```python
from build123d import *

# Parameters (mm, degrees)
POCKET003_DEPTH    = 10
POLARPATTERN_COUNT = 6


with BuildPart() as part:
    # Sketch012 → Revolution001 (revolve)
    with BuildSketch(Plane.XZ):
        Polygon((4, 0), (4, 2.040516), (7.084628, 2.040516), (7.084628, 14), (9, 14), (9, 0), align=None)
    revolve(axis=Axis((0, 0, 0), (0, 0, 1)))

    # Sketch013 → Pocket003 (cut, symmetric)
    with BuildSketch(Plane.XZ):
        with BuildLine():
            ThreePointArc((11.928039, 6.425307), (10.121972, 8.231374), (8.315905, 6.425307))
            Line((8.315905, 6.425307), (8.315905, -3.082439))
            ThreePointArc((8.315905, -3.082439), (10.121972, -4.888506), (11.928039, -3.082439))
            Line((11.928039, 6.425307), (11.928039, -3.082439))
        make_face()
    pocket003 = extrude(amount=POCKET003_DEPTH, both=True, mode=Mode.SUBTRACT)

    # PolarPattern: Pocket003 ×6 about axis
    polarpattern_axis = Axis((0, 0, 0), (0, 0, 1))
    for i in range(1, POLARPATTERN_COUNT):
        add(pocket003.rotate(polarpattern_axis, i * 360 / POLARPATTERN_COUNT), mode=Mode.SUBTRACT)


with BuildPart() as part_1:
    # Body006 placement: moved
    add(part.part.moved(Location((0, 0, -34))))


solid = part_1.part
```
The listing builds one solid part. Answer for the finished solid, in the listing's coordinates (mm). A direction names the side the tool comes from. Round coordinates to 2 decimals unless told otherwise and drop trailing zeros. Loops run counter-clockwise (first coordinate to the right, second up) from the corner with the lowest first, then second, coordinate; pieces in that order, holes last.
Q1. Section D-D, the plane y = 4.75 is taken. Determine the outline of the cut face in (x, z), then the cut area to 3 significant figures.
Q2. Which of the six approach directions +Z, -Z, +X, -X, +Y, -Y give full straight-line access (tool end or side, diameter ignored) to faces 5 (the face through (-8.316, 0, -31)), 6 (the face through (-4.116, 7.226, -30.742)), 7 (the face through (8.316, 0, -31)), 8 (the face through (4.2, 7.178, -30.742))?
Q3. Section C-C, the plane y = 0 is taken. Determine the outline of the cut face in (x, z), then the cut area to 3 significant figures.
Q4. Section B-B, the plane z = -28.25 is taken. Determine the outline of the cut face in (x, y).
Q5. Find the intervals of material crossed by line 1 (Y direction, x = 0, z = -33.35); line 2 (Z direction, x = -6, y = -0.75); line 3 (Y direction, x = 6.5, z = -28.5), in increasing order.
Q6. For a pull along Y with two mould halves and no side action, classify faces 1 (the face through (-0.867, -3.905, -32.965)), 2 (the face through (-4.17, 7.33, -26.94)), 3 (the face through (-4.257, -7.277, -26.941)), 4 (the face through (-3, -3, -31.959)) as released by +Y, released by -Y, zero draft, split by the parting line, or undercut.
Q7. Section A-A, the plane x = 0 is taken. Determine the outline of the cut face in (y, z), then the cut area to 3 significant figures.
Q8. Given pin 1 Ø1.5 at (x, z) = (-4, -23) entering from +Y; pin 2 Ø7 at (y, z) = (-1.5, -31) entering from +X; pin 3 Ø1.5 at (y, z) = (2.5, -24) entering from +X, each flat-ended and moving along its own axis, determine where each tip first touches the part or whether it passes through.
Completed:
1. outline: (-7.64, -34) - (7.64, -34) - (7.64, -20) - (5.26, -20) - (5.26, -31.96) - (-5.26, -31.96) - (-5.26, -20) - (-7.64, -20) - close
1. area: 88.3 mm2
2. face 5: -Z, -X, +Y, -Y
2. face 6: -Z, -X, +Y
2. face 7: -Z, +X, +Y, -Y
2. face 8: -Z, +X, +Y
3. outline: (-9, -26.16) arc R1.81 cw to (-8.32, -27.57) - (-8.32, -34) - (-4, -34) - (-4, -31.96) - (-7.08, -31.96) - (-7.08, -20) - (-9, -20) - close; (4, -34) - (8.32, -34) - (8.32, -27.57) arc R1.81 cw to (9, -26.16) - (9, -20) - (7.08, -20) - (7.08, -31.96) - (4, -31.96) - close
3. area: 56.1 mm2
4. outline: (-8.32, -3.44) arc R9 ccw to (-7.14, -5.48) - (-1.18, -8.92) arc R9 ccw to (1.18, -8.92) - (7.14, -5.48) arc R9 ccw to (8.32, -3.44) - (8.32, 3.44) arc R9 ccw to (7.14, 5.48) - (1.18, 8.92) arc R9 ccw to (-1.18, 8.92) - (-7.14, 5.48) arc R9 ccw to (-8.32, 3.44) - close; hole circle Ø14.17 at (0, 0)
5. line 1: y = -9 to -4, 4 to 9
5. line 2: z = -34 to -31.96
5. line 3: y = -5.85 to -2.82, 2.82 to 5.85
6. face 1: undercut
6. face 2: released by +Y
6. face 3: released by -Y
6. face 4: undercut
7. outline: (-9, -34) - (-4, -34) - (-4, -31.96) - (-7.08, -31.96) - (-7.08, -20) - (-9, -20) - close; (4, -34) - (9, -34) - (9, -20) - (7.08, -20) - (7.08, -31.96) - (4, -31.96) - close
7. area: 66.2 mm2
8. pin 1: stops at y = 8.39
8. pin 2: stops at x = 8.32
8. pin 3: stops at x = 8.83
